CAD build for the part. Positions are in the model's coordinates, mm. A direction names the side the tool comes from. Round coordinates to 2 decimals unless told otherwise and drop trailing zeros. Loops run counter-clockwise (first coordinate to the right, second up) from the corner with the lowest first, then second, coordinate; pieces in that order, holes last.
from build123d import *

# Parameters (mm, degrees)
BOSS_EXTRUDE1_DEPTH   = 48
HOLE1_D               = 10
BOSS_EXTRUDE2_DEPTH   = 2
CIRPATTERN1_COUNT     = 6
HOLE2_D               = 15
CIRPATTERN2_OUTLINE_R = 7.5
CIRPATTERN2_DEPTH     = 10


# Read off the part's stored shape, not the designer's step: CirPattern2
with BuildPart() as part:
    # Sketch1 → Revolve1 (revolve)
    with BuildSketch(Plane.XY, mode=Mode.PRIVATE) as revolve1_sk:
        Polygon((12, 0), (12, 10), (13, 10), (18, 20), (18, 75), (30, 75), (30, 10), (60, 10), (60, 0), align=None)
    revolve(revolve1_sk.sketch.rotate(Axis((0, 0, 0), (0, 1, 0)), 90), axis=Axis((0, 0, 0), (0, 1, 0)))

    # Sketch2 → Boss-Extrude1 (add)
    with BuildSketch(Plane.XY.offset(24)):
        with BuildLine():
            Line((-20, 60), (-20, 40))
            ThreePointArc((-20, 40), (-35, 25), (-50, 40))
            Line((-50, 40), (-50, 60))
            ThreePointArc((-50, 60), (-45.606601718, 70.606601718), (-35, 75))
            Line((-35, 75), (-20, 75))
            Line((-20, 75), (-20, 60))
        make_face()
    extrude(amount=-BOSS_EXTRUDE1_DEPTH)

    # Hole1 (through all)
    with Locations(Plane.XY.offset(24)):
        with Locations((-38, 63), (-38, 39)):
            Hole(HOLE1_D / 2)

    # Sketch5 → Boss-Extrude2 (add, symmetric)
    with BuildSketch(Plane(origin=(0, 0, 0), x_dir=(0, 0, -1), z_dir=(1, 0, 0))):
        Polygon((28, 40), (50, 10), (28, 10), align=None)
    boss_extrude2 = extrude(amount=BOSS_EXTRUDE2_DEPTH, both=True)

    # CirPattern1: Boss-Extrude2 ×6 about axis
    cirpattern1_axis = Axis((0, 0, 0), (0, 1, 0))
    for i in range(1, CIRPATTERN1_COUNT):
        add(boss_extrude2.rotate(cirpattern1_axis, i * 360 / CIRPATTERN1_COUNT))

    # Hole2 (through all)
    with Locations(Plane(origin=(0, 10, 0), x_dir=(1, 0, 0), z_dir=(0, 1, 0))):
        with Locations((47.5, 0)):
            Hole(HOLE2_D / 2)

    # CirPattern2 outline → CirPattern2 (cut)
    with BuildSketch(Plane(origin=(0, 0, 0), x_dir=(1, 0, 0), z_dir=(0, 1, 0))):
        with Locations((23.75, 41.13620668)):
            Circle(CIRPATTERN2_OUTLINE_R)
        with Locations((-23.75, 41.13620668)):
            Circle(CIRPATTERN2_OUTLINE_R)
        with Locations((-47.5, 0)):
            Circle(CIRPATTERN2_OUTLINE_R)
        with Locations((-23.75, -41.13620668)):
            Circle(CIRPATTERN2_OUTLINE_R)
        with Locations((23.75, -41.13620668)):
            Circle(CIRPATTERN2_OUTLINE_R)
    extrude(amount=CIRPATTERN2_DEPTH, mode=Mode.SUBTRACT)


solid = part.part
Item 1: Mould opens along X. For faces 5 (the flat face through (2, 18, -36)), 6 (the cylindrical face through (40.346, 4.93, -2.253)), 7 (the flat face through (-35, 50, 24)) say: released by +X, released by -X, zero draft, split by the parting line, or undercut.
Verdict:
face 5: released by +X
face 6: undercut
face 7: zero draft
Item 2: Cut at D-D (y = 13.5). List the corners of the cut face in (x, z), plus the area to 3 significant figures.
Verdict:
outline: (-42.08, -21.98) - (-40.08, -25.45) - (-24.92, -16.7) arc R30 ccw to (-2, -29.93) - (-2, -47.43) - (2, -47.43) - (2, -29.93) arc R30 ccw to (24.92, -16.7) - (40.08, -25.45) - (42.08, -21.98) - (26.92, -13.23) arc R30 ccw to (26.92, 13.23) - (42.08, 21.98) - (40.08, 25.45) - (24.92, 16.7) arc R30 ccw to (2, 29.93) - (2, 47.43) - (-2, 47.43) - (-2, 29.93) arc R30 ccw to (-24.92, 16.7) - (-40.08, 25.45) - (-42.08, 21.98) - (-26.92, 13.23) arc R30 ccw to (-26.92, -13.23) - close; hole circle Ø29.5 at (0, 0)
area: 2,560 mm2
Item 3: Cut at A-A (y = 61.5). List the corners of the cut face in (x, z).
Verdict:
outline: (-49.92, -24) - (-42.77, -24) - (-42.77, 24) - (-49.92, 24) - close; (-33.23, -24) - (-20, -24) - (-20, -22.36) arc R30 ccw (long way) to (-20, 22.36) - (-20, 24) - (-33.23, 24) - close; hole circle Ø36 at (0, 0)
Item 4: 3-axis set-ups, long thin cutter, end or side, ignore diameter. For faces 1 (the flat face through (-2, 18, 36)), 2 (the flat face through (2, 18, 36)), 3 (the cylindrical face through (-12.165, 47.885, 13.267)), 4 (the flat face through (-35, 50, -24)): which of +Z, -Z, +X, -X, +Y, -Y reach the whole face in a straight line?
Verdict:
face 1: +Z, -X, +Y
face 2: +Z, +X, +Y
face 3: +Y
face 4: -Z, -X, +Y
Item 5: Wall check: L1, parallel to Z at x = 23, y = 7; L2, parallel to Z at x = -31, y = 58.5; L3, parallel to Y at x = -37, z = -23.5. Give the ranges that are in metal, low to high.
Verdict:
L1: z = -55.42 to -48.6, -33.67 to 33.67, 48.6 to 55.42
L2: z = -24 to 24
L3: y = 0 to 18.46, 25.13 to 34.1, 43.9 to 58.1, 67.9 to 74.87
Item 6: Flat gauge pins, fed straight in: P1, Ø19.5, axis at x = 23.75, z = 41.14, coming from the +Y side; P2, Ø6, axis at y = 64.5, z = -10.5, coming from the -X side; P3, Ø1, axis at x = -13.5, y = 36, coming from the -Z side; P4, Ø12, axis at x = -23.75, z = 41.14, coming from the -Y side. Where does each tip first touch, or does it go through?
Verdict:
P1: stops at y = 10
P2: stops at x = -49.92
P3: stops at z = -27.04
P4: passes through
Item 7: Cut at C-C (x = 0). List the corners of the cut face in (y, z), plus the area to 3 significant figures.
Verdict:
outline: (0, -60) - (10, -60) - (10, -50) - (37.27, -30) - (75, -30) - (75, -18) - (20, -18) - (10, -13) - (10, -12) - (0, -12) - close; (0, 12) - (10, 12) - (10, 13) - (20, 18) - (75, 18) - (75, 30) - (37.27, 30) - (10, 50) - (10, 60) - (0, 60) - close
area: 3,120 mm2
Item 8: Cut at B-B (x = -38). List the corners of the cut face in (y, z).
Verdict:
outline: (0, -46.43) - (10, -46.43) - (10, -24.25) - (16.77, -24.25) - (19.92, -19.63) - (10, -19.63) - (10, 19.63) - (19.92, 19.63) - (16.77, 24.25) - (10, 24.25) - (10, 46.43) - (0, 46.43) - close; (25.3, -24) - (34, -24) - (34, 24) - (25.3, 24) - close; (44, -24) - (58, -24) - (58, 24) - (44, 24) - close; (68, -24) - (74.7, -24) - (74.7, 24) - (68, 24) - close
